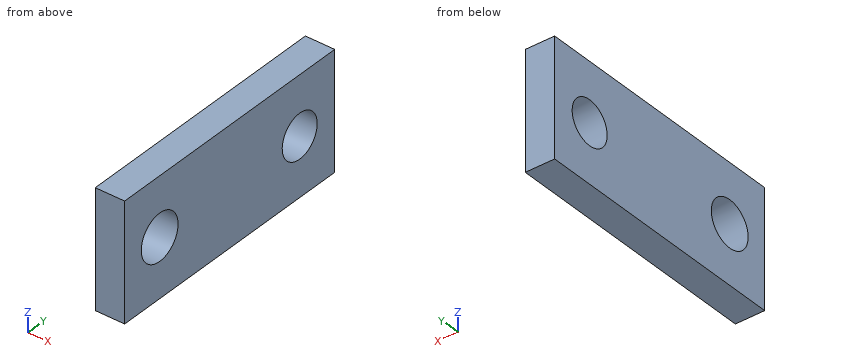
Autodesk Inventor part; units mm, degrees
ref_plane "YZ Plane" through (0, 0, 0) normal (1, 0, 0) x (0, 1, 0)
ref_plane "XZ Plane" through (0, 0, 0) normal (0, 1, 0) x (-1, 0, 0)
ref_plane "XY Plane" through (0, 0, 0) normal (0, 0, 1) x (1, 0, 0)
sketch "Sketch1" plane through (0, 0, 0) normal (1, 0, 0) x (0, 1, 0)
  line L0 (0, 0) -> (90, 0)
  line L1 (90, 0) -> (90, -40)
  line L2 (90, -40) -> (0, -40)
  line L3 (0, -40) -> (0, 0)
  dimension "d0" = 90
  dimension "d1" = 40
extrude "Extrusion1" add sketch "Sketch1" along normal blind 10
sketch "Sketch2" plane through (0, 0, 0) normal (-1, 0, 0) x (0, 0, 1)
  circle A0 centre (-20, 15) radius 7.8823
  line L0 (0, 0) -> (-40, 0)
  dimension "d4" = 15
extrude "Extrusion2" cut sketch "Sketch2" against normal mid plane 50
sketch "Sketch3" plane through (0, 0, 0) normal (-1, 0, 0) x (0, 0, 1)
  circle A0 centre (-20, 75) radius 7.5
  line L0 (-40, 90) -> (0, 90)
  point P0 (0, 0)
  dimension "d7" = 15
  dimension "d8" = 15
extrude "Extrusion3" cut sketch "Sketch3" against normal mid plane 50
properties part number "holder"
Work out the finished part from the listing and answer in its coordinate system (mm). Give positions to 0.01 mm unless a question says otherwise; leave off trailing zeros. Order: outer loops, then holes, each group sorted by start corner. A loop starts at its lowest first (then second) coordinate and runs counter-clockwise, first axis right, second up. Notation, with made-up numbers: M 56.25,43.25 L 64.25,43.25 A15 ccw 64.25,59.25 Z; hole C -24,43.25 d4. An arc over 180 degrees is marked long. Return JSON: item names as keys, results as strings.
Q1. Find section C-C, the plane y = 75. Write down the section's boundary in (x, z).
Answer below:
{"outline": "M 0,-40 L 10,-40 L 10,-27.5 L 0,-27.5 Z; M 0,-12.5 L 10,-12.5 L 10,0 L 0,0 Z"}
Q2. Find section A-A, the plane y = 15. Write down the section's boundary in (x, z).
Answer below:
{"outline": "M 0,-40 L 10,-40 L 10,-27.88 L 0,-27.88 Z; M 0,-12.12 L 10,-12.12 L 10,0 L 0,0 Z"}
Q3. Find section B-B, the plane z = -20. Write down the section's boundary in (x, y).
Answer below:
{"outline": "M 0,0 L 10,0 L 10,7.12 L 0,7.12 Z; M 0,22.88 L 10,22.88 L 10,67.5 L 0,67.5 Z; M 0,82.5 L 10,82.5 L 10,90 L 0,90 Z"}
Q4. Find section D-D, the plane x = 3.5. Write down the section's boundary in (y, z).
Answer below:
{"outline": "M 0,-40 L 90,-40 L 90,0 L 0,0 Z; hole C 15,-20 d15.76; hole C 75,-20 d15"}
Q5. This flat-tipped pin is pushed along its axis until it touches: pin 1 (10 mm diameter, centred on y = 45.5, z = -7, fed in from -X). Where does it stop, or does it pass through?
Answer below:
{"pin 1": "stops at x = 0"}
Q6. Find the intervals of material crossed by line 1 along Y through (x, z) = (5.25, -20); line 2 along Y through (x, z) = (9, -24); line 3 along Z through (x, y) = (2.25, 70), in increasing order. Write a range as [from, to].
Answer below:
{"line 1": "y = [0, 7.12], [22.88, 67.5], [82.5, 90]", "line 2": "y = [0, 8.21], [21.79, 68.66], [81.34, 90]", "line 3": "z = [-40, -25.59], [-14.41, 0]"}
